Geometry: see drawing. Coordinates: mm, zero at the bounding-box minimum. Round coordinates to 2 decimals unless told otherwise and drop trailing zeros. Order: outer loops, then holes, each group sorted by start corner. A loop starts at its lowest first (then second) coordinate and runs counter-clockwise, first axis right, second up. Notation, with made-up numbers: M 87.5,76 L 111.5,76 A27 ccw 111.5,115 Z; hole C 13.25,21 d8. An arc over 180 degrees is marked long. Answer in a Markdown table with one row per item. Add a question column.
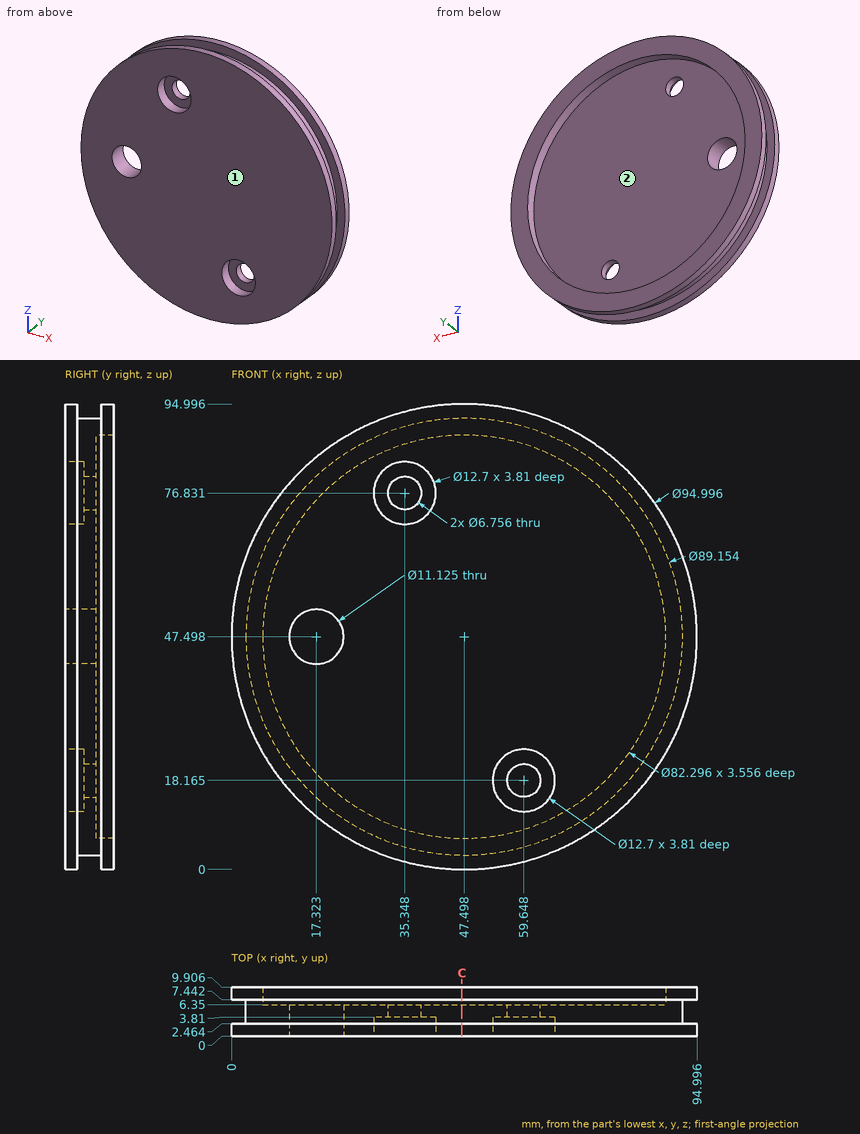
(1) Draft query along X for the marked faces 1 and 2. Return one class per face: +X half, -X half, draft (parallel to the pull), parting line (faces both ways), or undercut.
(2) Line query: line 1 (Y direction, x = 12, z = 19.5); line 2 (Y direction, x = 31.5, z = 52.5). Output: solid intervals per line, ascending. Write a range as from..to.
(3) Pin query (flat end, axial travel): pin 1 (5.5 mm diameter, centred on x = 35.35, z = 76.83, fed in from +Y); pin 2 (6.5 mm diameter, centred on x = 34.5, z = 78, fed in from -Y); pin 3 (1 mm diameter, centred on x = 44.5, y = 1, fed in from +Z); pin 4 (3 mm diameter, centred on x = 17, z = 53, fed in from +Y). Return the tip coordinate at first contact, or that it passes through.
(4) Cut plane C-C (x = 47). Return loops of the section in (y, z), and give its area (3 significant figures).
Answer list:
| question | item | result |
|---|---|---|
| 1 | face 1 | draft |
| 1 | face 2 | undercut |
| 2 | line 1 | 0..2.46, 7.44..9.91 |
| 2 | line 2 | 0..6.35 |
| 3 | pin 1 | through |
| 3 | pin 2 | y = 3.81 |
| 3 | pin 3 | z = 94.93 |
| 3 | pin 4 | y = 6.35 |
| 4 | outline | M 0,0 L 2.46,0 L 2.46,2.92 L 7.44,2.92 L 7.44,0 L 9.91,0 L 9.91,6.35 L 6.35,6.35 L 6.35,88.64 L 9.91,88.64 L 9.91,94.99 L 7.44,94.99 L 7.44,92.07 L 2.46,92.07 L 2.46,94.99 L 0,94.99 Z |
| 4 | area | 619 mm² |
